Source: CAD feature listing. Evaluate the final solid. Frame: model axes, mm. A direction names the side the tool comes from. Round coordinates to 2 decimals unless told otherwise and drop trailing zeros. Write each loop counter-clockwise with the first axis right and the second up, starting at its lowest first coordinate (ties: lowest second). Pieces come first, ordered by that corner, then holes.
from build123d import *

# Parameters (mm, degrees)
F0_R     = 55
F0_R_2   = 1.6
F0_R_3   = 2.9
F1_DEPTH = 5
F2_R     = 10
F3_DEPTH = 10
F4_R     = 2.9
F5_DEPTH = 10
F6_R     = 2.5
F7_DEPTH = 10
F8_R     = 6
F8_R_2   = 5
F9_DEPTH = 1.5


with BuildPart() as f1:
    # F0 (on Top) → F1 (new body)
    with BuildSketch(Plane.XY):
        Circle(F0_R)
        with Locations((-17.320508, -10)):
            Circle(F0_R_2, mode=Mode.SUBTRACT)
        with Locations((17.320508, -10)):
            Circle(F0_R_2, mode=Mode.SUBTRACT)
        Circle(F0_R_3, mode=Mode.SUBTRACT)
        with Locations((0, 18.7)):
            Circle(F0_R_2, mode=Mode.SUBTRACT)
    extrude(amount=F1_DEPTH)

    # F2 (on face) → F3 (join)
    with BuildSketch(Plane(origin=(0, 0, 0), x_dir=(1, 0, 0), z_dir=(0, 0, -1))):
        Circle(F2_R)
    extrude(amount=F3_DEPTH)

    # F4 (on face) → F5 (cut)
    with BuildSketch(Plane.XY.offset(5)):
        Circle(F4_R)
    extrude(amount=-F5_DEPTH, mode=Mode.SUBTRACT)

    # F6 (on face) → F7 (join)
    with BuildSketch(Plane(origin=(0, 0, -10), x_dir=(1, 0, 0), z_dir=(0, 0, -1))):
        Circle(F6_R)
    extrude(amount=F7_DEPTH)

    # F8 (on face) → F9 (cut)
    with BuildSketch(Plane(origin=(0, 0, 0), x_dir=(1, 0, 0), z_dir=(0, 0, -1))):
        with Locations((-17.320508, 10)):
            Circle(F8_R)
        with Locations((17.320508, 10)):
            Circle(F8_R)
        with Locations((0, -18.7)):
            Circle(F8_R_2)
    extrude(amount=-F9_DEPTH, mode=Mode.SUBTRACT)


solid = f1.part
1) Section query D-D on z = -2.75. Return the cut outline in (x, y), then the cut area to 3 significant figures.
Taken from the geometry:
outline: circle Ø20 at (0, 0); hole circle Ø5.8 at (0, 0)
area: 288 mm2
2) Contact query for flat-ended pins moving along their axis: P1, Ø7, axis at x = 17.32, y = -10, coming from the +Z side; P2, Ø5, axis at x = 30.5, y = -35, coming from the -Z side; P3, Ø3.5, axis at x = -17.32, y = -10, coming from the -Z side; P4, Ø10, axis at x = -35.5, z = 0.5, coming from the -Y side. Output: stop coordinate, or through.
Taken from the geometry:
P1: stops at z = 5
P2: stops at z = 0
P3: stops at z = 1.5
P4: stops at y = -45.77
3) Section query A-A on x = 0. Return the cut outline in (y, z).
Taken from the geometry:
outline: (-55, 0) - (-10, 0) - (-10, -10) - (-2.5, -10) - (-2.5, -20) - (2.5, -20) - (2.5, -10) - (10, -10) - (10, 0) - (13.7, 0) - (13.7, 1.5) - (17.1, 1.5) - (17.1, 5) - (2.9, 5) - (2.9, -5) - (-2.9, -5) - (-2.9, 5) - (-55, 5) - close; (20.3, 1.5) - (23.7, 1.5) - (23.7, 0) - (55, 0) - (55, 5) - (20.3, 5) - close
4) Section query B-B on y = 0. Return the cut outline in (x, z), then the cut area to 3 significant figures.
Taken from the geometry:
outline: (-55, 0) - (-10, 0) - (-10, -10) - (-2.5, -10) - (-2.5, -20) - (2.5, -20) - (2.5, -10) - (10, -10) - (10, 0) - (55, 0) - (55, 5) - (2.9, 5) - (2.9, -5) - (-2.9, -5) - (-2.9, 5) - (-55, 5) - close
area: 742 mm2
5) Pull-direction query (X, two-part tool) for faces 4 (the face through (-11.923, -53.692, 2.465)), 5 (the face through (19, -9, 1.5)), 6 (the face through (0, 0, -20)), 7 (the face through (-22.082, -6.349, 0.74)); classes: released by +X, released by -X, zero draft, split by the parting line, or undercut.
Taken from the geometry:
face 4: split by the parting line
face 5: undercut
face 6: zero draft
face 7: undercut
6) Material intervals for line 1 (Y direction, x = 0, z = 4.05); line 2 (Z direction, x = 36.5, y = -39); line 3 (X direction, y = 18.7, z = 1.25), sorted ascending.
Taken from the geometry:
line 1: y = -55 to -2.9, 2.9 to 17.1, 20.3 to 55
line 2: z = 0 to 5
line 3: x = -51.72 to -5, 5 to 51.72
7) Reachability of faces 1 (the face through (2, 2, -10)), 2 (the face through (0, 0, -5)), 3 (the face through (18.06, -11.42, 3.23)) from +Z, -Z, +X, -X, +Y, -Y: full face, straight path, thin tool, end or side. Return the list, or none.
Taken from the geometry:
face 1: -Z
face 2: +Z
face 3: +Z, -Z
8) Section query C-C on y = 18.7. Return the cut outline in (x, z).
Taken from the geometry:
outline: (-51.72, 0) - (-5, 0) - (-5, 1.5) - (-1.6, 1.5) - (-1.6, 5) - (-51.72, 5) - close; (1.6, 1.5) - (5, 1.5) - (5, 0) - (51.72, 0) - (51.72, 5) - (1.6, 5) - close
